Design review of the part shown in the three views and the two pictorial views. Dimensions are in mm from the part's minimum x, y and z. Round coordinates to 2 decimals unless told otherwise and drop trailing zeros. Loops run counter-clockwise (first coordinate to the right, second up) from the corner with the lowest first, then second, coordinate; pieces in that order, holes last. Notation, with made-up numbers: M -25,24 L 16,24 A20 ccw 16,32 Z; hole C -22,79.5 d5. An arc over 180 degrees is marked long. Return JSON: item names as keys, results as strings. Group by question number.
Q1. To check wall thickness, follow line 1 along X through (y, z) = (273.5, 21.5); line 2 along X through (y, z) = (326.5, 26.5). State the ranges of each line that lie inside material, in increasing order.
Q2. Clearance check with flat-ended pins moving along their axes: pin 1 Ø20.5 at (x, z) = (1041, 11) entering from +Y (3 decimals); pin 2 Ø6 at (y, z) = (42.5, 13.5) entering from +X. State where each tip first meets the part, or that it passes through.
Q3. Consider section A-A (y = 56.5). State the section outline as (x, z) points.
Q4. Consider section B-B (y = 314.5). State the section outline as (x, z) points.
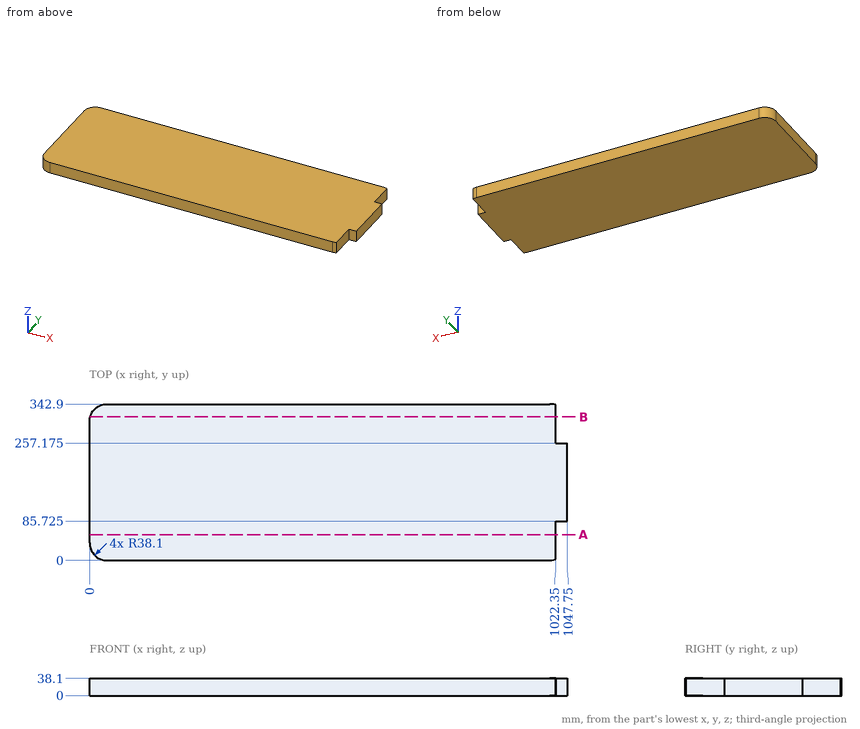
Values:
{
 "1": {"line 1": "x = 0 to 1022.35", "line 2": "x = 6.78 to 1022.35"},
 "2": {"pin 1": "stops at y = 257.175", "pin 2": "stops at x = 1022.35"},
 "3": {"outline": "M 0,0 L 1022.35,0 L 1022.35,38.1 L 0,38.1 Z"},
 "4": {"outline": "M 1.26,0 L 1022.35,0 L 1022.35,38.1 L 1.26,38.1 Z"}
}
